```python
from build123d import *

# Parameters (mm, degrees)
SKETCH1_R           = 1.7
BOSS_EXTRUDE3_DEPTH = 5
SKETCH5_W           = 78
SKETCH5_H           = 3.5
BOSS_EXTRUDE4_DEPTH = 10
SKETCH6_R           = 1.65
SKETCH6_R_2         = 1.7
CUT_EXTRUDE5_DEPTH  = 225.037103934
SKETCH8_R           = 1.65
CUT_EXTRUDE6_DEPTH  = 10
SKETCH9_R           = 1.7
CUT_EXTRUDE8_DEPTH  = 225.037103934


with BuildPart() as part:
    # Sketch1 → Boss-Extrude3 (new body)
    with BuildSketch(Plane(origin=(0, 0, 0), x_dir=(1, 0, 0), z_dir=(0, 1, 0))):
        Polygon((137.5, 44.585264028), (137.5, 5.555589367), (149.554092402, 5.555589367), (179.554092402, 5.555589367), (179.554092402, 13.614938689), (154.554092402, 13.614938689), (149.554092402, 18.614938689), (149.554092402, 120.555589367), (154.554092402, 125.555589367), (179.554092402, 125.555589367), (179.554092402, 133.614938689), (149.554092402, 133.614938689), (137.5, 133.614938689), (137.5, 94.585264028), (127.5, 84.585264028), (37.5, 84.585264028), (17.045454545, 119.585264028), (-82.954545455, 119.585264028), (-82.954545455, 19.585264028), (17.045454545, 19.585264028), (37.5, 54.585264028), (127.5, 54.585264028), align=None)
        with Locations(Location((138.726505033, 65.770964076, 0), (0, 0, 270))):
            Circle(SKETCH1_R, mode=Mode.SUBTRACT)
        with Locations(Location((121.557258463, 63.486894852, 0), (0, 0, 270))):
            Circle(SKETCH1_R, mode=Mode.SUBTRACT)
        with Locations(Location((128.163819776, 79.497933157, 0), (0, 0, 270))):
            Circle(SKETCH1_R, mode=Mode.SUBTRACT)
        with Locations(Location((175.173925842, 9.585264028, 0), (0, 0, 270))):
            Circle(SKETCH1_R, mode=Mode.SUBTRACT)
        with Locations(Location((175.173925842, 129.585264028, 0), (0, 0, 90))):
            Circle(SKETCH1_R, mode=Mode.SUBTRACT)
        with BuildLine():
            Line((-79.802677261, 28.560822148), (-66.688486942, 43.661087452))
            ThreePointArc((-66.688486942, 43.661087452), (-61.892029486, 43.998720199), (-61.554396738, 39.202262743))
            Line((-61.554396738, 39.202262743), (-74.668587058, 24.101997439))
            ThreePointArc((-74.668587058, 24.101997439), (-79.465044514, 23.764364691), (-79.802677261, 28.560822148))
        make_face(mode=Mode.SUBTRACT)
        with BuildLine():
            Line((-79.802677261, 110.609705909), (-66.688486942, 95.509440605))
            ThreePointArc((-66.688486942, 95.509440605), (-61.892029486, 95.171807858), (-61.554396738, 99.968265314))
            Line((-61.554396738, 99.968265314), (-74.668587058, 115.068530618))
            ThreePointArc((-74.668587058, 115.068530618), (-79.465044514, 115.406163365), (-79.802677261, 110.609705909))
        make_face(mode=Mode.SUBTRACT)
        with BuildLine():
            Line((13.893586352, 110.609705909), (0.779396033, 95.509440605))
            ThreePointArc((0.779396033, 95.509440605), (-4.017061423, 95.171807858), (-4.354694171, 99.968265314))
            Line((-4.354694171, 99.968265314), (8.759496149, 115.068530618))
            ThreePointArc((8.759496149, 115.068530618), (13.555953605, 115.406163365), (13.893586352, 110.609705909))
        make_face(mode=Mode.SUBTRACT)
        with BuildLine():
            Line((13.893586352, 28.560822148), (0.779396033, 43.661087452))
            ThreePointArc((0.779396033, 43.661087452), (-4.017061423, 43.998720199), (-4.354694171, 39.202262743))
            Line((-4.354694171, 39.202262743), (8.759496149, 24.101997439))
            ThreePointArc((8.759496149, 24.101997439), (13.555953605, 23.764364691), (13.893586352, 28.560822148))
        make_face(mode=Mode.SUBTRACT)
    extrude(amount=BOSS_EXTRUDE3_DEPTH)

    # Sketch5 → Boss-Extrude4 (add)
    with BuildSketch(Plane(origin=(0, 5, 0), x_dir=(1, 0, 0), z_dir=(0, 1, 0))):
        with Locations((-32.885058048, 47.835264028)):
            Rectangle(SKETCH5_W, SKETCH5_H)
        with Locations((-32.885058048, 91.335264028)):
            Rectangle(SKETCH5_W, SKETCH5_H)
    extrude(amount=BOSS_EXTRUDE4_DEPTH)

    # Sketch6 → Cut-Extrude5 (cut, through all)
    with BuildSketch(Plane(origin=(0, 5, 0), x_dir=(1, 0, 0), z_dir=(0, 1, 0))):
        with Locations(Location((-32.954545455, 47.824855797, 0), (0, 0, 270))):
            Circle(SKETCH6_R)
        with Locations(Location((-32.954545455, 59.701124199, 0), (0, 0, 270))):
            Circle(SKETCH6_R_2)
        with Locations(Location((-12.954545455, 59.791818088, 0), (0, 0, 270))):
            Circle(SKETCH6_R_2)
        with Locations(Location((-52.954545455, 59.791818088, 0), (0, 0, 270))):
            Circle(SKETCH6_R_2)
        with Locations(Location((-32.954545455, 91.34567226, 0), (0, 0, 90))):
            Circle(SKETCH6_R)
        with Locations(Location((-12.954545455, 79.378709969, 0), (0, 0, 90))):
            Circle(SKETCH6_R_2)
        with Locations(Location((-32.954545455, 79.469403858, 0), (0, 0, 90))):
            Circle(SKETCH6_R_2)
        with Locations(Location((-52.954545455, 79.378709969, 0), (0, 0, 90))):
            Circle(SKETCH6_R_2)
    extrude(amount=-CUT_EXTRUDE5_DEPTH, mode=Mode.SUBTRACT)

    # Sketch8 → Cut-Extrude6 (cut)
    with BuildSketch(Plane(origin=(0, 15, 0), x_dir=(1, 0, 0), z_dir=(0, 1, 0))):
        with Locations(Location((-32.885058048, 47.835264028, 0), (0, 0, 270))):
            Circle(SKETCH8_R)
        with Locations(Location((-32.885058048, 91.335264028, 0), (0, 0, 260.261217373))):
            Circle(SKETCH8_R)
    extrude(amount=-CUT_EXTRUDE6_DEPTH, mode=Mode.SUBTRACT)

    # Sketch9 → Cut-Extrude8 (cut, through all)
    with BuildSketch(Plane(origin=(0, 5, 0), x_dir=(1, 0, 0), z_dir=(0, 1, 0))):
        with Locations(Location((-23.954545455, 34.585264028, 0), (0, 0, 270))):
            Circle(SKETCH9_R)
        with Locations(Location((-41.954545455, 34.585264028, 0), (0, 0, 90))):
            Circle(SKETCH9_R)
        with Locations(Location((-41.954545455, 104.585264028, 0), (0, 0, 270))):
            Circle(SKETCH9_R)
        with Locations(Location((-23.954545455, 104.585264028, 0), (0, 0, 90))):
            Circle(SKETCH9_R)
    extrude(amount=-CUT_EXTRUDE8_DEPTH, mode=Mode.SUBTRACT)


solid = part.part
```
Part model, mm, in its own coordinate system. A direction names the side the tool comes from. Round coordinates to 2 decimals unless told otherwise and drop trailing zeros. Order: outer loops, then holes, each group sorted by start corner. A loop starts at its lowest first (then second) coordinate and runs counter-clockwise, first axis right, second up. Notation, with made-up numbers: M 74.25,13 L 100.25,13 A18 ccw 100.25,29 Z; hole C 26,68.25 d11. An arc over 180 degrees is marked long. Answer in a Markdown table with one row per item. Add a question column.
Q1. Cut at B-B on y = 12.75. Give the cut face in (x, z).
Q2. Cut at C-C on x = -18. Give the cut face in (y, z).
Q3. Cut at A-A on x = 158. Give the cut face in (y, z), and give its area (3 significant figures).
Q4. 3-axis set-ups, long thin cutter, end or side, ignore diameter. For faces 4 (the face through (7.428, 2.465, -36.005)), 5 (the face through (-33.4, 9.9, -46.085)), 6 (the face through (83, 2, -84.585)), 7 (the face through (-33.4, 9.9, -49.585)): which of +Z, -Z, +X, -X, +Y, -Y reach the whole face in a straight line?
Q5. Wall check: L1, parallel to Z at x = -52, y = 7.75; L2, parallel to Z at x = -64, y = 4.5; L3, parallel to X at y = 3.5, z = -126.5. Give the ranges that are in metal, low to high. Write a range as from..to.
Q6. Mould opens along Z. For faces 1 (the face through (27.13, 2.46, -36.84)), 2 (the face through (2.1, 2.5, -107.4)), 3 (the face through (-82.955, 2, -70)) say: +Z half, -Z half, draft (parallel to the pull), parting line (faces both ways), or undercut.
Q7. Pin check, flat tips, straight feed: pin 1 (3 mm diameter, centred on x = 30.5, y = 2, fed in from +Z); pin 2 (4 mm diameter, centred on y = 2.5, z = -44.5, fed in from +X); pin 3 (5.5 mm diameter, centred on x = 128.16, z = -79.5, fed in from +Y). Stop position of each tip, or through.
Q8. Cut at D-D on z = -72. Give the cut face in (x, y), and give its area (3 significant figures).
Established:
| question | item | result |
|---|---|---|
| 1 | outline | M -71.89,-93.09 L 6.11,-93.09 L 6.11,-89.59 L -71.89,-89.59 Z; M -71.89,-49.59 L 6.11,-49.59 L 6.11,-46.09 L -71.89,-46.09 Z; hole C -32.89,-91.34 d3.3; hole C -32.89,-47.84 d3.3 |
| 2 | outline | M 0,-119.59 L 5,-119.59 L 5,-93.09 L 15,-93.09 L 15,-89.59 L 5,-89.59 L 5,-49.59 L 15,-49.59 L 15,-46.09 L 5,-46.09 L 5,-19.59 L 0,-19.59 Z |
| 3 | outline | M 0,-133.61 L 5,-133.61 L 5,-125.56 L 0,-125.56 Z; M 0,-13.61 L 5,-13.61 L 5,-5.56 L 0,-5.56 Z |
| 3 | area | 80.6 mm2 |
| 4 | face 4 | +Y, -Y |
| 4 | face 5 | +Z, +X, -X, +Y |
| 4 | face 6 | -Z, +Y, -Y |
| 4 | face 7 | +X, -X, +Y |
| 5 | L1 | z = -93.09..-89.59, -49.59..-46.09 |
| 5 | L2 | z = -119.59..-102.78, -94.34..-44.83, -36.39..-19.59 |
| 5 | L3 | x = 137.5..179.55 |
| 6 | face 1 | +Z half |
| 6 | face 2 | undercut |
| 6 | face 3 | draft |
| 7 | pin 1 | stops at z = -40.04 |
| 7 | pin 2 | stops at x = 149.55 |
| 7 | pin 3 | stops at y = 5 |
| 8 | outline | M -82.95,0 L 149.55,0 L 149.55,5 L -82.95,5 Z |
| 8 | area | 1,160 mm2 |
